Verification items for the finished model (mm, model axes). Give positions to 0.01 mm unless a question says otherwise; leave off trailing zeros. Order: outer loops, then holes, each group sorted by start corner. A loop starts at its lowest first (then second) coordinate and runs counter-clockwise, first axis right, second up. Notation, with made-up numbers: M 21.5,63 L 72.5,63 A33 ccw 72.5,94 Z; hole C 87,78.25 d6. An arc over 180 degrees is marked long. Answer as a JSON object with one key per item and string values.
```python
from build123d import *

# Parameters (mm, degrees)
F0_R     = 2.6
F1_DEPTH = 6


with BuildPart() as f1:
    # F0 (on Right) → F1 (new body)
    with BuildSketch(Plane.YZ):
        with BuildLine():
            Line((-50.484604, 0), (0, 0))
            Line((0, 0), (50.484604, 0))
            ThreePointArc((50.484604, 0), (50.854025, 0.013666), (51.221427, 0.054589))
            Line((51.221427, 0.054589), (123.236823, 10.784256))
            ThreePointArc((123.236823, 10.784256), (126.287091, 12.465017), (127.5, 15.729667))
            Line((127.5, 15.729667), (127.5, 32.709328))
            ThreePointArc((127.5, 32.709328), (126.139466, 36.137781), (122.798285, 37.700423))
            Line((122.798285, 37.700423), (51.004047, 41.991095))
            ThreePointArc((51.004047, 41.991095), (50.854971, 41.997773), (50.705762, 42))
            Line((50.705762, 42), (39.15917, 42))
            Line((39.15917, 42), (-39.15917, 42))
            Line((-39.15917, 42), (-50.705762, 42))
            ThreePointArc((-50.705762, 42), (-50.854971, 41.997773), (-51.004047, 41.991095))
            Line((-51.004047, 41.991095), (-122.798285, 37.700423))
            ThreePointArc((-122.798285, 37.700423), (-126.139466, 36.137781), (-127.5, 32.709328))
            Line((-127.5, 32.709328), (-127.5, 15.729667))
            ThreePointArc((-127.5, 15.729667), (-126.287091, 12.465017), (-123.236823, 10.784256))
            Line((-123.236823, 10.784256), (-51.221427, 0.054589))
            ThreePointArc((-51.221427, 0.054589), (-50.854025, 0.013666), (-50.484604, 0))
        make_face()
        with Locations((-121.5, 16.095773)):
            Circle(F0_R, mode=Mode.SUBTRACT)
        with Locations((121.5, 16.095773)):
            Circle(F0_R, mode=Mode.SUBTRACT)
        with BuildLine():
            Line((-50.855038, 30.681556), (-50.855038, 11.866378))
            ThreePointArc((-50.855038, 11.866378), (-52.590387, 8.079287), (-56.591861, 6.920966))
            Line((-56.591861, 6.920966), (-111.236823, 15.06259))
            ThreePointArc((-111.236823, 15.06259), (-114.287091, 16.743351), (-115.5, 20.008001))
            Line((-115.5, 20.008001), (-115.5, 27.415784))
            ThreePointArc((-115.5, 27.415784), (-114.139466, 30.844237), (-110.798285, 32.406879))
            Line((-110.798285, 32.406879), (-56.153323, 35.672651))
            ThreePointArc((-56.153323, 35.672651), (-52.426585, 34.321022), (-50.855038, 30.681556))
        make_face(mode=Mode.SUBTRACT)
        with Locations((-121.5, 31.328013)):
            Circle(F0_R, mode=Mode.SUBTRACT)
        with BuildLine():
            ThreePointArc((-39.855038, 6), (-43.390572, 7.464466), (-44.855038, 11))
            Line((-44.855038, 11), (-44.855038, 31))
            ThreePointArc((-44.855038, 31), (-43.390572, 34.535534), (-39.855038, 36))
            Line((-39.855038, 36), (-39.15917, 36))
            Line((-39.15917, 36), (39.15917, 36))
            Line((39.15917, 36), (39.855038, 36))
            ThreePointArc((39.855038, 36), (43.390572, 34.535534), (44.855038, 31))
            Line((44.855038, 31), (44.855038, 11))
            ThreePointArc((44.855038, 11), (43.390572, 7.464466), (39.855038, 6))
            Line((39.855038, 6), (0, 6))
            Line((0, 6), (-39.855038, 6))
        make_face(mode=Mode.SUBTRACT)
        with BuildLine():
            Line((56.153323, 35.672651), (110.798285, 32.406879))
            ThreePointArc((110.798285, 32.406879), (114.139466, 30.844237), (115.5, 27.415784))
            Line((115.5, 27.415784), (115.5, 20.008001))
            ThreePointArc((115.5, 20.008001), (114.287091, 16.743351), (111.236823, 15.06259))
            Line((111.236823, 15.06259), (56.591861, 6.920966))
            ThreePointArc((56.591861, 6.920966), (52.590387, 8.079287), (50.855038, 11.866378))
            Line((50.855038, 11.866378), (50.855038, 30.681556))
            ThreePointArc((50.855038, 30.681556), (52.426585, 34.321022), (56.153323, 35.672651))
        make_face(mode=Mode.SUBTRACT)
        with Locations((121.5, 31.328013)):
            Circle(F0_R, mode=Mode.SUBTRACT)
    extrude(amount=F1_DEPTH)


solid = f1.part
```
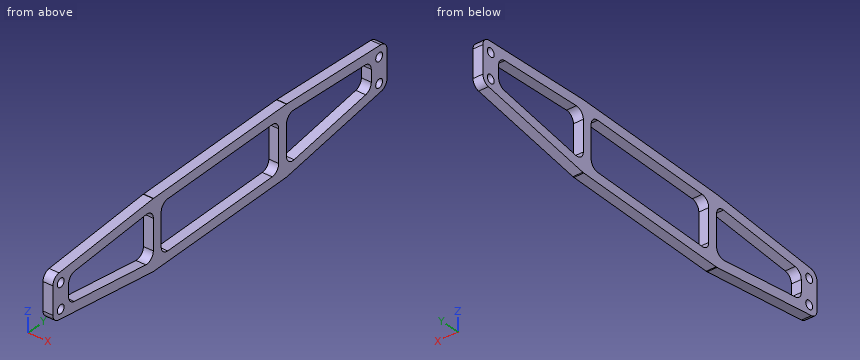
Q1. Section check C-C on x = 2.65. Count the separate pieces of the cut face and the enclosed holes in it, then the cut area to 3 significant figures.
Resolved:
{"separate pieces": "1", "enclosed holes": "7", "area": "3,760 mm²"}
Q2. Gauge pin test, flat ends, axial feed: pin 1 Ø1 at (x, z) = (3.5, 34) entering from +Y; pin 2 Ø4 at (y, z) = (-121.5, 31.33) entering from -X; pin 3 Ø1 at (x, z) = (5, 36.5) entering from -Y. Record the tip position at first contact, or that the pin passes through.
Resolved:
{"pin 1": "stops at y = 127.44", "pin 2": "passes through", "pin 3": "stops at y = -126.26"}
Q3. Section check B-B on y = -33. Record the cut outline in (x, z).
Resolved:
{"outline": "M 0,0 L 6,0 L 6,6 L 0,6 Z; M 0,36 L 6,36 L 6,42 L 0,42 Z"}
Q4. Section check A-A on z = 23. Record the cut outline in (x, y).
Resolved:
{"outline": "M 0,-127.5 L 6,-127.5 L 6,-115.5 L 0,-115.5 Z; M 0,-50.86 L 6,-50.86 L 6,-44.86 L 0,-44.86 Z; M 0,44.86 L 6,44.86 L 6,50.86 L 0,50.86 Z; M 0,115.5 L 6,115.5 L 6,127.5 L 0,127.5 Z"}
Q5. Material ranges on L1, parallel to Y at x = 3.9, z = 26.5; L2, parallel to Z at x = 3.05, y = 121.5; L3, parallel to Y at x = 1.3, z = 17.5, recorded low to high.
Resolved:
{"L1": "y = -127.5 to -115.5, -50.86 to -44.86, 44.86 to 50.86, 115.5 to 127.5", "L2": "z = 10.53 to 13.5, 18.7 to 28.73, 33.93 to 37.78", "L3": "y = -127.5 to -123.69, -119.31 to -114.83, -50.86 to -44.86, 44.86 to 50.86, 114.83 to 119.31, 123.69 to 127.5"}
